```python
from build123d import *

# Parameters (mm, degrees)
SKETCH_1_R      = 2.65
SKETCH_1_R_2    = 1.6
EXTRUDE_1_DEPTH = 3


with BuildPart() as part:
    # 草图1 → 凸台-拉伸1 (new body)
    with BuildSketch(Plane(origin=(0, 0, 0), x_dir=(1, 0, 0), z_dir=(0, 1, 0))):
        Polygon((-15.222569187, 19.831121687), (14.743614759, 21.25513704), (69.57570845, 23.860798923), (71.474395588, -16.094113005), (16.642301897, -18.699774888), (-13.323882049, -20.123790241), align=None)
        with Locations((-0.0496085, 16.547638171)):
            Circle(SKETCH_1_R, mode=Mode.SUBTRACT)
        with Locations((1.46934121, -15.416291372)):
            Circle(SKETCH_1_R, mode=Mode.SUBTRACT)
        with Locations((-8.994058556, -5.902235174)):
            Circle(SKETCH_1_R_2, mode=Mode.SUBTRACT)
        with Locations((-9.563664698, 6.084238404)):
            Circle(SKETCH_1_R_2, mode=Mode.SUBTRACT)
        with Locations((10.413791266, 7.033581973)):
            Circle(SKETCH_1_R_2, mode=Mode.SUBTRACT)
        with Locations((10.983397408, -4.952891605)):
            Circle(SKETCH_1_R_2, mode=Mode.SUBTRACT)
        with Locations((62.773467577, 19.533037481)):
            Circle(SKETCH_1_R, mode=Mode.SUBTRACT)
        with Locations((64.292417287, -12.430892061)):
            Circle(SKETCH_1_R, mode=Mode.SUBTRACT)
    extrude(amount=EXTRUDE_1_DEPTH)


solid = part.part
```
Source: CAD feature listing. Evaluate the final solid. Frame: model axes, mm. Round coordinates to 2 decimals unless told otherwise and drop trailing zeros. Loops run counter-clockwise (first coordinate to the right, second up) from the corner with the lowest first, then second, coordinate; pieces in that order, holes last. Notation, with made-up numbers: M 76,23.25 L 91,23.25 A28 ccw 91,47.25 Z; hole C 75,8.5 d7. An arc over 180 degrees is marked long. Use a Markdown table: item, result. Add a question column.
1. Mould query, pull axis Z, two halves, no side actions, for faces 1 (the flat face through (29, 0, -2)), 2 (the cylindrical face through (62.189, 1.479, 14.043)), 3 (the flat face through (70.51, 1.48, -4.16)). Classes: pulls with the +Z half, pulls with the -Z half, needs draft (parallel to the pull), parting line crosses it, or undercut.
2. Section query A-A on z = -18. Return the cut outline in (x, y), then the cut area to 3 significant figures.
3. Section query B-B on y = 1.6. Give the number of separate pieces and of enclosed holes in the cut face, then the cut area to 3 significant figures.
4. Section query D-D on z = -12. Return the cut outline in (x, y).
5. Line query: line 1 (X direction, y = 1.6, z = 6); line 2 (X direction, y = 2.75, z = -17.5); line 3 (Z direction, x = 3, y = 2.8). Output: solid intervals per line, ascending.
6. Section query C-C on z = 17. Return the cut outline in (x, y), then the cut area to 3 significant figures.
7. Contact query for flat-ended pins moving along their axis: P1, Ø1.5, axis at y = 2.5, z = 5.5, coming from the -X side; P2, Ø2.5, axis at x = -8.99, z = 5.9, coming from the +Y side; P3, Ø1, axis at y = 2.5, z = -2, coming from the -X side. Output: stop coordinate, or through.
Reported:
| question | item | result |
|---|---|---|
| 1 | face 1 | needs draft |
| 1 | face 2 | undercut |
| 1 | face 3 | pulls with the -Z half |
| 2 | outline | M -15.14,0 L -2.27,0 L -2.27,3 L -15.14,3 Z; M 2.17,0 L 60.61,0 L 60.61,3 L 2.17,3 Z; M 64.94,0 L 69.85,0 L 69.85,3 L 64.94,3 Z |
| 2 | area | 229 mm² |
| 3 | separate pieces | 1 |
| 3 | enclosed holes | 8 |
| 3 | area | 3,280 mm² |
| 4 | outline | M -14.85,0 L 70.14,0 L 70.14,3 L -14.85,3 Z |
| 5 | line 1 | x = -14 to -10.59, -7.4 to 9.77, 12.19 to 70.99 |
| 5 | line 2 | x = -15.11 to -2.52, 2.42 to 61.07, 64.47 to 69.88 |
| 5 | line 3 | z = -20.7 to 13.25, 17.58 to 19.35 |
| 6 | outline | M -13.47,0 L -0.66,0 L -0.66,3 L -13.47,3 Z; M 3.59,0 L 52.41,0 L 52.41,3 L 3.59,3 Z |
| 6 | area | 185 mm² |
| 7 | P1 | stops at x = -14.05 |
| 7 | P2 | passes through |
| 7 | P3 | stops at x = -14.4 |
